from build123d import *

# Parameters (mm, degrees)
EXTRUDE_1_DEPTH          = 5
SKETCH_2_R               = 2.1
CUT_EXTRUDE_1_DEPTH      = 6
PATTERN_CIRCULAR_1_COUNT = 3
SKETCH_3_R               = 2.1
CUT_EXTRUDE_2_DEPTH      = 6
PATTERN_CIRCULAR_2_COUNT = 3
SKETCH_4_R               = 2.1
CUT_EXTRUDE_3_DEPTH      = 6
PATTERN_CIRCULAR_3_COUNT = 3
FILLET_1_R               = 50
SKETCH_5_R               = 5
CUT_EXTRUDE_4_DEPTH      = 1
CUT_EXTRUDE_4_DEPTH_BACK = 6


with BuildPart() as part:
    # 草图1 → 凸台-拉伸1 (new body)
    with BuildSketch(Plane(origin=(0, 0, 0), x_dir=(1, 0, 0), z_dir=(0, 1, 0))):
        Polygon((57.735026919, 100), (-57.735026919, 100), (-115.470053838, 0), (-57.735026919, -100), (57.735026919, -100), (115.470053838, 0), align=None)
    extrude(amount=EXTRUDE_1_DEPTH)

    # 草图2 → 切除-拉伸1 (cut, through all)
    with BuildSketch(Plane(origin=(0, 5, 0), x_dir=(1, 0, 0), z_dir=(0, 1, 0))):
        with Locations((-23.5, 37)):
            Circle(SKETCH_2_R)
        with Locations((23.5, 37)):
            Circle(SKETCH_2_R)
        with Locations((-23.5, 63)):
            Circle(SKETCH_2_R)
        with Locations((23.5, 63)):
            Circle(SKETCH_2_R)
        with Locations((-23.5, 89)):
            Circle(SKETCH_2_R)
        with Locations((23.5, 89)):
            Circle(SKETCH_2_R)
    cut_extrude_1 = extrude(amount=-CUT_EXTRUDE_1_DEPTH, mode=Mode.SUBTRACT)

    # 阵列(圆周)1: 切除-拉伸1 ×3 about axis
    pattern_circular_1_axis = Axis((0, 0, 0), (0, 1, 0))
    for i in range(1, PATTERN_CIRCULAR_1_COUNT):
        add(cut_extrude_1.rotate(pattern_circular_1_axis, i * 360 / PATTERN_CIRCULAR_1_COUNT), mode=Mode.SUBTRACT)

    # 草图3 → 切除-拉伸2 (cut, through all)
    with BuildSketch(Plane(origin=(0, 5, 0), x_dir=(1, 0, 0), z_dir=(0, 1, 0))):
        with Locations((65.326260937, 64.851596989)):
            Circle(SKETCH_3_R)
        with Locations((88.826260937, 24.148403011)):
            Circle(SKETCH_3_R)
        with Locations((54.559600438, 31.5)):
            Circle(SKETCH_3_R)
    cut_extrude_2 = extrude(amount=-CUT_EXTRUDE_2_DEPTH, mode=Mode.SUBTRACT)

    # 阵列(圆周)2: 切除-拉伸2 ×3 about axis
    pattern_circular_2_axis = Axis((0, 0, 0), (0, 1, 0))
    for i in range(1, PATTERN_CIRCULAR_2_COUNT):
        add(cut_extrude_2.rotate(pattern_circular_2_axis, i * 360 / PATTERN_CIRCULAR_2_COUNT), mode=Mode.SUBTRACT)

    # 草图4 → 切除-拉伸3 (cut, through all)
    with BuildSketch(Plane(origin=(0, 5, 0), x_dir=(1, 0, 0), z_dir=(0, 1, 0))):
        with Locations((0, 20)):
            Circle(SKETCH_4_R)
    cut_extrude_3 = extrude(amount=-CUT_EXTRUDE_3_DEPTH, mode=Mode.SUBTRACT)

    # 阵列(圆周)3: 切除-拉伸3 ×3 about axis
    pattern_circular_3_axis = Axis((0, 0, 0), (0, 1, 0))
    for i in range(1, PATTERN_CIRCULAR_3_COUNT):
        add(cut_extrude_3.rotate(pattern_circular_3_axis, i * 360 / PATTERN_CIRCULAR_3_COUNT), mode=Mode.SUBTRACT)

    # 圆角1
    fillet_1_edges = [part.edges().sort_by_distance(p)[0] for p in [
        (115.470053838, 2.5, 0),
        (57.735026919, 2.5, 100),
        (-57.735026919, 2.5, 100),
        (-115.470053838, 2.5, 0),
        (-57.735026919, 2.5, -100),
        (57.735026919, 2.5, -100),
    ]]
    fillet(fillet_1_edges, radius=FILLET_1_R)

    # 草图5 → 切除-拉伸4 (cut, two sides)
    with BuildSketch(Plane(origin=(0, 5, 0), x_dir=(1, 0, 0), z_dir=(0, 1, 0))) as cut_extrude_4_sk:
        Circle(SKETCH_5_R)
    extrude(amount=CUT_EXTRUDE_4_DEPTH, mode=Mode.SUBTRACT)
    extrude(cut_extrude_4_sk.sketch, amount=-CUT_EXTRUDE_4_DEPTH_BACK, mode=Mode.SUBTRACT)


solid = part.part
Input: part model. Units: mm. Frame: model coordinates. Coordinates: 2 decimals unless noted, no trailing zeros. Loops run counter-clockwise (first coordinate to the right, second up) from the corner with the lowest first, then second, coordinate; pieces in that order, holes last. Notation, with made-up numbers: (38.25, 68) -> (78.25, 68) arc R29 cw to (78.25, 107) -> close; hole circle Ø6 at (-11.5, 87). An arc over 180 degrees is marked (long way). One line per item, written item: value.
(1) Cut plane C-C (z = -84). Output: boundary loops of the cut face in (x, y), then the cut area to 3 significant figures.
Answer below:
outline: (-65.53, 0) -> (65.53, 0) -> (65.53, 5) -> (-65.53, 5) -> close
area: 655 mm2
(2) Cut plane B-B (y = 2). Give the number of separate pieces and of enclosed holes in the cut face, then the cut area to 3 significant figures.
Answer below:
separate pieces: 1
enclosed holes: 31
area: 33,300 mm2
(3) Ray query, line 1 along Z through (x, y) = (23, 1.75); line 2 along X through (y, z) = (1.95, 53); line 3 along X through (y, z) = (1.95, -63). Return the intervals inside material, ascending.
Answer below:
line 1: z = -100 to -91.04, -86.96 to -65.04, -60.96 to -39.04, -34.96 to 86.96, 91.04 to 100
line 2: x = -84.87 to -44.57, -41.05 to 41.05, 44.57 to 84.87
line 3: x = -79.1 to -66.32, -64.34 to -25.6, -21.4 to 21.4, 25.6 to 64.34, 66.32 to 79.1
(4) Draft query along Z for faces 1 (the face through (-107.734, 2.535, -0.367)), 2 (the face through (-54.18, 2.54, 93.12)), 3 (the face through (-1.08, 2.54, 4.88)). Return one class per face: pulls with the +Z half, pulls with the -Z half, needs draft (parallel to the pull), parting line crosses it, or undercut.
Answer below:
face 1: parting line crosses it
face 2: pulls with the +Z half
face 3: undercut
(5) Cut plane A-A (z = -56.5). Output: boundary loops of the cut face in (x, y).
Answer below:
outline: (-82.85, 0) -> (82.85, 0) -> (82.85, 5) -> (-82.85, 5) -> close
(6) Pin query (flat end, axial travel): pin 1 Ø5.5 at (x, z) = (88.83, 24.15) entering from -Y; pin 2 Ø1.5 at (y, z) = (3.5, -49.5) entering from -X; pin 3 Ø3 at (x, y) = (-74.5, 4.5) entering from +Z; pin 4 Ø1.5 at (y, z) = (3, -28.5) entering from +X. Return the tip coordinate at first contact, or that it passes through.
Answer below:
pin 1: stops at y = 0
pin 2: stops at x = -87.32
pin 3: stops at z = 73.56
pin 4: stops at x = 99.45
